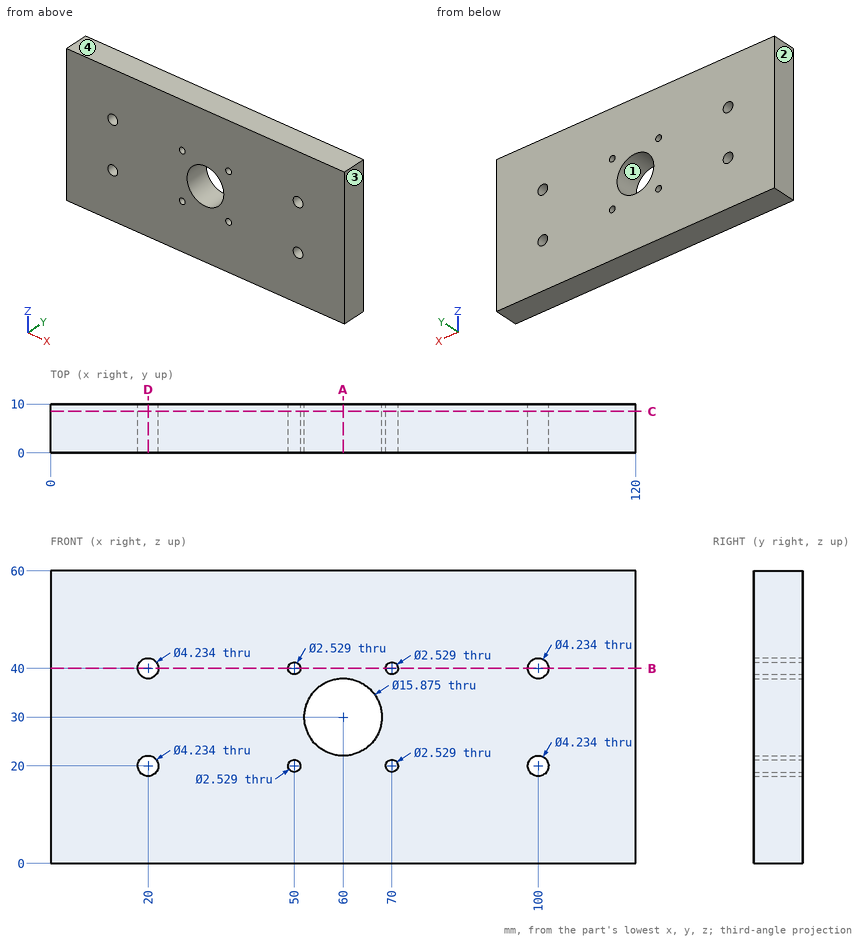
The drawing under review shows one solid part. Ordinate dimensions are in mm from its lowest x, y, z. Coordinates: 2 decimals unless noted, no trailing zeros. Order: outer loops, then holes, each group sorted by start corner. A loop starts at its lowest first (then second) coordinate and runs counter-clockwise, first axis right, second up. Notation, with made-up numbers: (86.25, -28.75) - (127.25, -28.75) arc R11 ccw to (127.25, -8.75) - close; hole circle Ø2 at (68, 15.5). An arc over 180 degrees is marked (long way). Put each result on its own line as item: value.
1) Insertion check: P1, Ø3.5, axis at x = 70, z = 20, coming from the -Y side; P2, Ø4, axis at x = 20, z = 40, coming from the -Y side. Each pin has a flat end and moves straight along its axis. Give the tip position at first contact, or say it passes through.
Response values:
P1: stops at y = 0
P2: passes through
2) Take a section at B-B, the plane z = 40. Give the boundary of the cut face in (x, y), and give its area (3 significant figures).
Response values:
outline: (0, 0) - (17.88, 0) - (17.88, 10) - (0, 10) - close; (22.12, 0) - (48.74, 0) - (48.74, 10) - (22.12, 10) - close; (51.26, 0) - (68.74, 0) - (68.74, 10) - (51.26, 10) - close; (71.26, 0) - (97.88, 0) - (97.88, 10) - (71.26, 10) - close; (102.12, 0) - (120, 0) - (120, 10) - (102.12, 10) - close
area: 1,060 mm²
3) Take a section at D-D, the plane x = 20. Give the boundary of the cut face in (y, z).
Response values:
outline: (0, 0) - (10, 0) - (10, 17.88) - (0, 17.88) - close; (0, 22.12) - (10, 22.12) - (10, 37.88) - (0, 37.88) - close; (0, 42.12) - (10, 42.12) - (10, 60) - (0, 60) - close
4) Take a section at A-A, the plane x = 60. Give the boundary of the cut face in (y, z), and give its area (3 significant figures).
Response values:
outline: (0, 0) - (10, 0) - (10, 22.06) - (0, 22.06) - close; (0, 37.94) - (10, 37.94) - (10, 60) - (0, 60) - close
area: 441 mm²
5) Take a section at C-C, the plane y = 8.5. Count the separate pieces of the cut face and the enclosed holes in it, and give its area (3 significant figures).
Response values:
separate pieces: 1
enclosed holes: 9
area: 6,930 mm²
6) Wall thickness on L1, parallel to Z at x = 50, y = 3; L2, parallel to Z at x = 100, y = 5.25; L3, parallel to X at y = 5, z = 40: over which ranges is each line inside the solid? List them lowest first. Write a range as from..to.
Response values:
L1: z = 0..18.74, 21.26..38.74, 41.26..60
L2: z = 0..17.88, 22.12..37.88, 42.12..60
L3: x = 0..17.88, 22.12..48.74, 51.26..68.74, 71.26..97.88, 102.12..120
7) The part is to be moulded in two halves that separate along X. For the marked faces 1, 2, 3 and 4, say which applies: released by +X, released by -X, zero draft, split by the parting line, or undercut.
Response values:
face 1: undercut
face 2: released by -X
face 3: released by +X
face 4: zero draft
